Input: part model. Units: mm. Frame: model coordinates. Coordinates: 2 decimals unless noted, no trailing zeros. Write each loop counter-clockwise with the first axis right and the second up, starting at its lowest first coordinate (ties: lowest second). Pieces come first, ordered by that corner, then holes. Notation, with made-up numbers: (84, -22) -> (124, -22) arc R16 ccw to (124, 5) -> close; hole circle Ø3 at (83.25, 76). An arc over 180 degrees is marked (long way). Use one line per item in the form item = value. Start each with the question number.
(1) Cut plane C-C on z = 0.15. Return the cut outline in (x, y), plus the area to 3 significant figures.
(2) Cut plane B-B on x = 77.5. Return the cut outline in (y, z), plus the area to 3 significant figures.
(3) Cut plane A-A on y = 2. Return the cut outline in (x, z).
(4) Ray query, line 1 along Y through (x, z) = (88.5, 0.6); line 2 along X through (y, z) = (18, 0.6); line 3 along Y through (x, z) = (66.5, 0.7). Return the intervals inside material, ascending.
(5) First-contact query: pin 1 (3 mm diameter, centred on x = -88.5, y = 47.25, fed in from +Z) (1 decimal). Flat tip, straight axial feed; report the tip coordinate or a pass-through.
Autodesk Fusion 360 part; units mm, degrees
sketch "Sketch1" plane through (0, 0, 0) normal (0, 0, 1) x (1, 0, 0)
  line L0 (88.5, -47.25) -> (-88.5, -47.25) construction
  line L1 (-88.5, -47.25) -> (-88.5, 47.25) construction
  line L2 (-88.5, 47.25) -> (88.5, 47.25) construction
  line L3 (88.5, 47.25) -> (88.5, -47.25) construction
  line L4 (88.5, -47.25) -> (-88.5, 47.25) construction
  line L5 (-88.5, -47.25) -> (88.5, 47.25) construction
  circle A0 centre (-88.5, 47.25) radius 1.75
  circle A1 centre (88.5, 47.25) radius 1.75
  circle A2 centre (88.5, -47.25) radius 1.75
  circle A3 centre (-88.5, -47.25) radius 1.75
  circle A4 centre (88.5, -47.25) radius 2.5
  circle A5 centre (88.5, 47.25) radius 2.5
  circle A6 centre (-88.5, 47.25) radius 2.5
  circle A7 centre (-88.5, -47.25) radius 2.5
  line L6 (86, -47.25) -> (-86, -47.25)
  line L7 (-86, -47.25) -> (-86, 47.25)
  line L8 (-86, 47.25) -> (86, 47.25)
  line L9 (86, 47.25) -> (86, -47.25)
  line L10 (86, -47.25) -> (-86, 47.25) construction
  line L11 (-86, -47.25) -> (86, 47.25) construction
  line L12 (99, -57.5) -> (-116, -57.5)
  line L13 (-116, -57.5) -> (-116, 57.5)
  line L14 (-116, 57.5) -> (99, 57.5)
  line L15 (99, 57.5) -> (99, -57.5)
  dimension "d1" = 177
  dimension "d2" = 94.5
  dimension "d3" = 3.5
  dimension "d4" = 3.5
  dimension "d5" = 3.5
  dimension "d6" = 3.5
  dimension "d7" = 5
  dimension "d8" = 5
  dimension "d9" = 5
  dimension "d10" = 5
  dimension "d11" = 215
  dimension "d12" = 115
  dimension "d15" = 27.5
  dimension "d16" = 57.5
extrude "Extrude1" add sketch "Sketch1" along normal blind 1 contours A4 | A7 | A6 | A5 | L12 L13 L14 L15
sketch "Sketch2" plane through (0, 0, 1) normal (0, 0, 1) x (-1, 0, 0)
  circle A0 centre (-88.5, -47.25) radius 1.75
  circle A1 centre (88.5, -47.25) radius 1.75
  line L0 (86, -47.25) -> (-86, -47.25)
  line L1 (-86, -47.25) -> (-86, 47.25)
  line L2 (-86, 47.25) -> (86, 47.25)
  line L3 (86, 47.25) -> (86, -47.25)
  circle A2 centre (88.5, 47.25) radius 1.75
  circle A3 centre (-88.5, 47.25) radius 1.75
  line L4 (-99, -57.5) -> (116, -57.5)
  line L5 (116, -57.5) -> (116, 57.5)
  line L6 (116, 57.5) -> (-99, 57.5)
  line L7 (-99, 57.5) -> (-99, -57.5)
Values:
q1.outline = (-116, -57.5) -> (99, -57.5) -> (99, 57.5) -> (-116, 57.5) -> close; hole circle Ø3.5 at (-88.5, -47.25); hole circle Ø3.5 at (-88.5, 47.25); hole (-86, -47.25) -> (86, -47.25) -> (86, 47.25) -> (-86, 47.25) -> close; hole circle Ø3.5 at (88.5, -47.25); hole circle Ø3.5 at (88.5, 47.25)
q1.area = 8,430 mm2
q2.outline = (-57.5, 0) -> (-47.25, 0) -> (-47.25, 1) -> (-57.5, 1) -> close; (47.25, 0) -> (57.5, 0) -> (57.5, 1) -> (47.25, 1) -> close
q2.area = 20.5 mm2
q3.outline = (-116, 0) -> (-86, 0) -> (-86, 1) -> (-116, 1) -> close; (86, 0) -> (99, 0) -> (99, 1) -> (86, 1) -> close
q4.line_1 = -57.5 to -49, -45.5 to 45.5, 49 to 57.5
q4.line_2 = -116 to -86, 86 to 99
q4.line_3 = -57.5 to -47.25, 47.25 to 57.5
q5.pin_1 = through
